```python
from build123d import *

# Parameters (mm, degrees)
F1_DEPTH = 2.38125
F2_R     = 2.38125
F3_DEPTH = 25.4
F5_DEPTH = 25.4


# Not quite as in the source:
# - a length typed as a fraction of an inch, garbled in the dataset ("3 / 203.2 mm" for 3/8 in), is restored


with BuildPart() as f1:
    # F0 (on Front) → F1 (new body)
    with BuildSketch(Plane.XZ):
        with BuildLine():
            Line((60.325, 19.05), (7.9502, 19.05))
            ThreePointArc((7.9502, 19.05), (2.3285596682, 16.7214403318), (0, 11.0998))
            Line((0, 11.0998), (0, 0))
            Line((0, 0), (9.525, 0))
            Line((9.525, 0), (11.7155767468, 7.5558858532))
            ThreePointArc((11.7155767468, 7.5558858532), (13.1960389642, 9.7526651699), (15.6788970925, 10.6762577523))
            Line((15.6788970925, 10.6762577523), (60.325, 12.7))
            Line((60.325, 12.7), (60.325, 19.05))
        make_face()
    extrude(amount=F1_DEPTH)

    # F2 (on face) → F3 (cut)
    with BuildSketch(Plane.XZ.offset(2.38125)):
        with Locations((7.9375, 11.1125)):
            Circle(F2_R)
    extrude(amount=-F3_DEPTH, mode=Mode.SUBTRACT)

    # F4 (on face) → F5 (cut)
    with BuildSketch(Plane.XY.offset(19.05)):
        Polygon((60.325, 0), (45.24375, 0), (60.325, -0.79375), align=None)
        Polygon((60.325, -2.38125), (60.325, -1.5875), (45.24375, -2.38125), align=None)
    extrude(amount=-F5_DEPTH, mode=Mode.SUBTRACT)


solid = f1.part
```
Can you work these out from the model? Positions are in its coordinate system, mm. Round coordinates to 2 decimals unless told otherwise and drop trailing zeros. Loops run counter-clockwise (first coordinate to the right, second up) from the corner with the lowest first, then second, coordinate; pieces in that order, holes last. Notation, with made-up numbers: M 43.25,35 L 101.25,35 A18 ccw 101.25,51 Z; hole C 50.5,50 d6. An arc over 180 degrees is marked long. Answer as a JSON object with one key per item and string values. Group by question number.
Q1. Please list where these lines run through material, in increasing order: L1, parallel to Z at x = 8.5, y = -2.2; L2, parallel to Z at x = 38.5, y = -2; L3, parallel to Z at x = 45.5, y = -1.25.
Q2. Imagine slicing it at A-A, the plane z = 9.5. Please give me the cut outline in (x, y), then the cut area to 3 significant figures.
Q3. We'd pull the mould along Z, two halves only. Please class faces 1 (the flat face through (10.605, -1.174, 3.725)), 2 (the flat face through (35, -1, 19.05)), 3 (the cylindrical face through (6.18, -1.21, 12.72)), 4 (the flat face through (17, -2.381, 12)): +Z half, -Z half, draft (parallel to the pull), parting line (faces both ways), or undercut.
Q4. Imagine slicing it at B-B, the plane z = 17.25. Please give me the cut outline in (x, y) (1 decimal).
Q5. Imagine slicing it at C-C, the plane x = 42.5. Please give me the cut outline in (y, z), then the cut area to 3 significant figures.
Q6. Imagine slicing it at D-D, the plane x = 20. Please give me the cut outline in (y, z).
Findings:
{
 "1": {"L1": "z = 0 to 8.8, 13.43 to 19.05", "L2": "z = 11.71 to 19.05", "L3": "z = 12.03 to 19.05"},
 "2": {"outline": "M 0,-2.38 L 6.19,-2.38 L 6.19,0 L 0,0 Z; M 9.69,-2.38 L 12.9,-2.38 L 12.9,0 L 9.69,0 Z", "area": "22.4 mm2"},
 "3": {"face 1": "-Z half", "face 2": "+Z half", "face 3": "undercut", "face 4": "draft"},
 "4": {"outline": "M 2.9,-2.4 L 45.2,-2.4 L 60.3,-1.6 L 60.3,-0.8 L 45.2,0 L 2.9,0 Z"},
 "5": {"outline": "M -2.38,11.89 L 0,11.89 L 0,19.05 L -2.38,19.05 Z", "area": "17.0 mm2"},
 "6": {"outline": "M -2.38,10.87 L 0,10.87 L 0,19.05 L -2.38,19.05 Z"}
}
